```python
from build123d import *

# Parameters (mm, degrees)
F1_DEPTH       = 3
F3_DEPTH       = 30
F4_W           = 29
F4_H           = 37
F5_DEPTH       = 33.001
F6_W           = 32.2
F6_H           = 40.2
F7_DEPTH       = 1.5
F9_DEPTH       = 22
F10_W          = 16.1
F10_H          = 8
F11_DEPTH      = 20
F13_DEPTH      = 53.501
F13_DEPTH_BACK = 16.501
F15_DEPTH      = 57.501
F17_DEPTH      = 12.5
F19_DEPTH      = 12.5
F20_R          = 0.5
F21_R          = 1


with BuildPart() as f1:
    # F0 (on Top) → F1 (new body)
    with BuildSketch(Plane.XY):
        with BuildLine():
            Line((-25, -35), (25, -35))
            ThreePointArc((25, -35), (32.0710678119, -32.0710678119), (35, -25))
            Line((35, -25), (35, 25))
            ThreePointArc((35, 25), (32.0710678119, 32.0710678119), (25, 35))
            Line((25, 35), (-25, 35))
            ThreePointArc((-25, 35), (-32.0710678119, 32.0710678119), (-35, 25))
            Line((-35, 25), (-35, -25))
            ThreePointArc((-35, -25), (-32.0710678119, -32.0710678119), (-25, -35))
        make_face()
    extrude(amount=F1_DEPTH)

    # F2 (on face) → F3 (join)
    with BuildSketch(Plane.XY.offset(3)):
        with BuildLine():
            Line((-16.5, -22.5), (16.5, -22.5))
            ThreePointArc((16.5, -22.5), (17.9142135624, -21.9142135624), (18.5, -20.5))
            Line((18.5, -20.5), (18.5, 20.5))
            ThreePointArc((18.5, 20.5), (17.9142135624, 21.9142135624), (16.5, 22.5))
            Line((16.5, 22.5), (-16.5, 22.5))
            ThreePointArc((-16.5, 22.5), (-17.9142135624, 21.9142135624), (-18.5, 20.5))
            Line((-18.5, 20.5), (-18.5, -20.5))
            ThreePointArc((-18.5, -20.5), (-17.9142135624, -21.9142135624), (-16.5, -22.5))
        make_face()
    extrude(amount=F3_DEPTH)

    # F4 (on face) → F5 (cut, through all)
    with BuildSketch(Plane.XY.offset(33)):
        Rectangle(F4_W, F4_H)
    extrude(amount=-F5_DEPTH, mode=Mode.SUBTRACT)

    # F6 (on face) → F7 (cut)
    with BuildSketch(Plane.XY.offset(33)):
        Rectangle(F6_W, F6_H)
    extrude(amount=-F7_DEPTH, mode=Mode.SUBTRACT)

    # F8 (on face) → F9 (cut)
    with BuildSketch(Plane.XY.offset(31.5)):
        Polygon((16.1, 20.1), (12.1, 20.1), (12.1, 18.5), (14.5, 18.5), (14.5, 3.1), (16.1, 3.1), align=None)
    extrude(amount=-F9_DEPTH, mode=Mode.SUBTRACT)

    # F10 (on face) → F11 (cut)
    with BuildSketch(Plane.XY.offset(33)):
        with Locations((-8.05, -16.1)):
            Rectangle(F10_W, F10_H)
    extrude(amount=-F11_DEPTH, mode=Mode.SUBTRACT)

    # F12 (on face) → F13 (cut, two sides)
    with BuildSketch(Plane.YZ.offset(18.5)) as f13_sk:
        with BuildLine():
            Line((-5, 8.030303205), (5, 8.030303205))
            ThreePointArc((5, 8.030303205), (8.5355339059, 9.4947692991), (10, 13.030303205))
            Line((10, 13.030303205), (10, 23.030303205))
            ThreePointArc((10, 23.030303205), (8.5355339059, 26.5658371109), (5, 28.030303205))
            Line((5, 28.030303205), (-5, 28.030303205))
            ThreePointArc((-5, 28.030303205), (-8.5355339059, 26.5658371109), (-10, 23.030303205))
            Line((-10, 23.030303205), (-10, 13.030303205))
            ThreePointArc((-10, 13.030303205), (-8.5355339059, 9.4947692991), (-5, 8.030303205))
        make_face()
    extrude(amount=-F13_DEPTH, mode=Mode.SUBTRACT)
    extrude(f13_sk.sketch, amount=F13_DEPTH_BACK, mode=Mode.SUBTRACT)

    # F14 (on face) → F15 (cut, through all)
    with BuildSketch(Plane.XZ.offset(22.5)):
        with BuildLine():
            Line((-5, 33), (-5, 23))
            ThreePointArc((-5, 23), (-0.0284616664, 18.0000810073), (4.9996759734, 22.9430775894))
            Line((4.9996759734, 22.9430775894), (5.114176247, 33))
            Line((5.114176247, 33), (-5, 33))
        make_face()
    extrude(amount=-F15_DEPTH, mode=Mode.SUBTRACT)

    # F16 (on face) → F17 (join, through all)
    with BuildSketch(Plane.XZ.offset(22.5)):
        Polygon((-16.5, 15.9740547451), (-16.5, 3), (16.5, 3), (16.5, 15.9740547451), (0, 18), align=None)
    extrude(amount=F17_DEPTH)

    # F18 (on face) → F19 (join, through all)
    with BuildSketch(Plane(origin=(0, 22.5, 0), x_dir=(-1, 0, 0), z_dir=(0, 1, 0))):
        Polygon((-16.5, 15.9741357524), (-16.5, 3), (16.5, 3), (16.5, 15.9741357524), (0, 18.0000810073), align=None)
    extrude(amount=F19_DEPTH)

    # F20
    f20_edges = [f1.edges().sort_by_distance(p)[0] for p in [
        (5.114176, -21.3, 33),
        (10.607088, -20.1, 33),
        (16.1, 0, 33),
        (10.607088, 20.1, 33),
        (5.114176, 21.3, 33),
        (10.807088, 22.5, 33),
        (17.914214, 21.914214, 33),
        (18.5, 0, 33),
        (17.914214, -21.914214, 33),
        (10.807088, -22.5, 33),
        (-17.914214, -21.914214, 33),
        (-18.5, 0, 33),
        (-17.914214, 21.914214, 33),
        (-10.75, 22.5, 33),
        (-5, 21.3, 33),
        (-10.55, 20.1, 33),
        (-16.1, 0, 33),
        (-10.55, -20.1, 33),
        (-5, -21.3, 33),
        (-10.75, -22.5, 33),
        (14.5, -7.7, 31.5),
        (9.798549, -18.5, 31.5),
        (-14.5, 3.2, 31.5),
        (-9.75, 18.5, 31.5),
        (8.598549, 18.5, 31.5),
    ]]
    fillet(f20_edges, radius=F20_R)

    # F21
    f21_edges = [f1.edges().sort_by_distance(p)[0] for p in [
        (16.5, 28.75, 3),
        (8.25, 35, 16.987108),
        (-8.25, 35, 16.987108),
        (-16.5, 28.75, 3),
        (-16.5, 35, 9.487068),
        (16.5, 35, 9.487068),
        (18.5, 0, 3),
        (16.5, -28.75, 3),
        (-16.5, -28.75, 3),
        (-16.5, -35, 9.487027),
        (-16.5, 28.75, 15.974136),
        (-35, 0, 3),
        (-32.071068, 32.071068, 3),
        (-20.75, 35, 3),
        (-20.75, -35, 3),
        (-32.071068, -32.071068, 3),
        (20.75, 35, 3),
        (-16.5, -28.75, 15.974055),
        (16.5, -35, 9.487027),
        (20.75, -35, 3),
        (16.5, 28.75, 15.974136),
        (32.071068, 32.071068, 3),
        (35, 0, 3),
        (32.071068, -32.071068, 3),
        (17.914214, -21.914214, 3),
        (17.914214, 21.914214, 3),
        (16.5, -28.75, 15.974055),
    ]]
    fillet(f21_edges, radius=F21_R)


solid = f1.part
```
Can you work these out from the model? Positions are in its coordinate system, mm. A direction names the side the tool comes from. Coordinates: 2 decimals unless noted, no trailing zeros. Loops run counter-clockwise (first coordinate to the right, second up) from the corner with the lowest first, then second, coordinate; pieces in that order, holes last. Notation, with made-up numbers: (45.5, 74) -> (69.5, 74) arc R17 ccw to (69.5, 107) -> close; hole circle Ø2 at (52, 86). An arc over 180 degrees is marked (long way). Put each result on its own line as item: value. Start each with the question number.
Q1. For faces 4 (the face through (-16, 0, 8.03)), 5 (the face through (17.9, -21.93, 18.05)), 6 (the face through (0, 20, 18)), 7 (the face through (35, 0, 1)), 8 (the face through (-15, -12.1, 22)), which set-ups out of +Z, -Z, +X, -X, +Y, -Y let a thin tool reach every point of the face, with its end or its side?
Q2. I want a section at D-D (x = 20.5). Write out the boundary of the cut face in (y, z).
Q3. I want a section at B-B (y = -8). Count the separate pieces of the cut face and the enclosed holes in it, plus the area to 3 significant figures.
Q4. If I drill on line 1 (X direction, y = 11, z = 8.5); line 2 (Y direction, x = 2, z = 2.5); line 3 (Y direction, x = -12, z = 31), over which ranges is the centre line in solid material (lowest first)? Write a range as [from, to].
Q5. Thinking about a two-plate mould opening in Z: for faces 1 (the face through (-26, 0, 3)), 2 (the face through (-10, 22.5, 24)), 3 (the face through (16.53, -8.57, 9.53)), which applies, pulls with the +Z half, pulls with the -Z half, needs draft (parallel to the pull), parting line crosses it, or undercut?
Q6. I'm going to push flat-ended pins straight in: P1, Ø5, axis at x = 5, z = 25.5, coming from the +Y side; P2, Ø5, axis at x = 18.5, z = 12, coming from the -Y side; P3, Ø13, axis at x = 25.5, y = -13.5, coming from the +Z side; P4, Ø3, axis at x = -17, y = -2.5, coming from the -Z side. Where does each tip first touch, or does it pass through?
Taken from the geometry:
1. face 4: +X, -X
1. face 5: +Z, +X, -Y
1. face 6: +Z, +Y, -Y
1. face 7: +Z, -Z, +X, +Y, -Y
1. face 8: +Z
2. outline: (-35, 0) -> (35, 0) -> (35, 2) arc R1 ccw to (34, 3) -> (-34, 3) arc R1 ccw to (-35, 2) -> close
3. separate pieces: 4
3. enclosed holes: 0
3. area: 214 mm2
4. line 1: x = [-18.5, -14.5], [14.5, 18.5]
4. line 2: y = [-35, -18.5], [18.5, 35]
4. line 3: y = [-22.5, -20.1], [18.5, 22.5]
5. face 1: pulls with the +Z half
5. face 2: needs draft
5. face 3: undercut
6. P1: stops at y = 22.5
6. P2: stops at y = -34.87
6. P3: stops at z = 3.13
6. P4: stops at z = 0
